Design review of the part built by this model. Coordinates are the model's own, in mm. A direction names the side the tool comes from. Round coordinates to 2 decimals unless told otherwise and drop trailing zeros. Loops run counter-clockwise (first coordinate to the right, second up) from the corner with the lowest first, then second, coordinate; pieces in that order, holes last. Notation, with made-up numbers: (-18.5, 53) - (22.5, 53) arc R35 cw to (22.5, 90) - close; hole circle Ø3 at (6, 47.25). An arc over 180 degrees is marked (long way). Return JSON: item names as keys, results as strings. Group by question number.
from build123d import *

# Parameters (mm, degrees)
FILLET1_R      = 6
CHAMFER1_SIZE  = 1
CHAMFER1_SIZE2 = 2
CHAMFER2_SIZE  = 0.5


with BuildPart() as part:
    # Sketch1 → Revolve1 (revolve)
    with BuildSketch(Plane(origin=(0, 0, 0), x_dir=(0, 0, -1), z_dir=(1, 0, 0))):
        Polygon((0, 0), (0, -80), (11, -80), (11, -77), (2.5, -77), (2.5, -8), (1.5, -8), (1.5, -3), (2.5, -3), (2.5, 0), align=None)
    revolve(axis=Axis((0, 0, 0), (0, -1, 0)))

    # Fillet1
    fillet1_edges = [part.edges().sort_by_distance(p)[0] for p in [
        (0, -77, 2.5),
    ]]
    fillet(fillet1_edges, radius=FILLET1_R)

    # Chamfer1
    chamfer1_edges = [part.edges().sort_by_distance(p)[0] for p in [
        (0, -77, 11),
    ]]
    chamfer1_side = [part.faces().sort_by_distance(p)[0] for p in [
        (0, -77, 8.811126984),
    ]]
    chamfer(chamfer1_edges, length=CHAMFER1_SIZE, length2=CHAMFER1_SIZE2, reference=chamfer1_side[0])

    # Chamfer2
    chamfer2_edges = [part.edges().sort_by_distance(p)[0] for p in [
        (0, 0, 2.5),
    ]]
    chamfer(chamfer2_edges, length=CHAMFER2_SIZE)


solid = part.part
Q1. Add section A-A, the plane x = 0. State the section outline as (y, z) points.
Q2. Insertion check: pin 1 Ø10 at (y, z) = (-28, -4.5) entering from -X; pin 2 Ø1 at (y, z) = (-14, 3.5) entering from +X; pin 3 Ø6 at (x, y) = (-3.5, -21.5) entering from +Z; pin 4 Ø6 at (y, z) = (-14, -3.5) entering from +X. Each pin has a flat end and moves straight along its axis. Give the tip position at first contact, or say it passes through.
Q3. Add section D-D, the plane y = -73.5. State the section outline as (x, z) points.
Q4. Tool access review of faces 4 (the cylindrical face through (-2.44, -39.06, 0.54)), 5 (the cylindrical face through (0.07, -5.46, 1.5)), 6 (the cylindrical face through (-10.74, -79.49, 2.38)): name each direction out of +Z, -Z, +X, -X, +Y, -Y from which nothing blocks a thin tool from reaching the whole face with its end or side.
Q5. Add section C-C, the plane y = -28.5. State the section outline as (x, z) points, plus the area to 3 significant figures.
Q6. For line 1 (Y direction, x = 5.75, z = 6.75); line 2 (Z direction, x = -1.5, y = -67); line 3 (Z direction, x = 1.75, y = -11), list the stretches that pass through material, from the lowest coordinate up.
Q7. Add section B-B, the plane z = 0. State the section outline as (x, y) points.
Q8. Draft analysis for pull direction Y (two halves, no side actions). For faces 1 (the flat face through (0, -80, 0)), 2 (the flat face through (0, -3, 2)), 3 (the flat face through (-7.4, -77, 4.5)), state which applies: pulls with the +Y half, pulls with the -Y half, needs draft (parallel to the pull), parting line crosses it, or undercut.
Evaluation:
{
 "1": {"outline": "(-80, -11) - (-79, -11) - (-77, -10) - (-77, -8.5) arc R6 cw to (-71, -2.5) - (-8, -2.5) - (-8, -1.5) - (-3, -1.5) - (-3, -2.5) - (-0.5, -2.5) - (0, -2) - (0, 2) - (-0.5, 2.5) - (-3, 2.5) - (-3, 1.5) - (-8, 1.5) - (-8, 2.5) - (-71, 2.5) arc R6 cw to (-77, 8.5) - (-77, 10) - (-79, 11) - (-80, 11) - close"},
 "2": {"pin 1": "x = -2.5", "pin 2": "through", "pin 3": "z = 2.45", "pin 4": "x = 2.45"},
 "3": {"outline": "circle Ø6.09 at (0, 0)"},
 "4": {"face 4": "+Y", "face 5": "none", "face 6": "+Y, -Y"},
 "5": {"outline": "circle Ø5 at (0, 0)", "area": "19.6 mm²"},
 "6": {"line 1": "-80 to -77", "line 2": "-2 to 2", "line 3": "-1.79 to 1.79"},
 "7": {"outline": "(-11, -80) - (11, -80) - (11, -79) - (10, -77) - (8.5, -77) arc R6 cw to (2.5, -71) - (2.5, -8) - (1.5, -8) - (1.5, -3) - (2.5, -3) - (2.5, -0.5) - (2, 0) - (-2, 0) - (-2.5, -0.5) - (-2.5, -3) - (-1.5, -3) - (-1.5, -8) - (-2.5, -8) - (-2.5, -71) arc R6 cw to (-8.5, -77) - (-10, -77) - (-11, -79) - close"},
 "8": {"face 1": "pulls with the -Y half", "face 2": "undercut", "face 3": "pulls with the +Y half"}
}
